Design review of the part built by this model. Coordinates are the model's own, in mm. A direction names the side the tool comes from. Coordinates: 2 decimals unless noted, no trailing zeros. Write each loop counter-clockwise with the first axis right and the second up, starting at its lowest first coordinate (ties: lowest second). Pieces come first, ordered by that corner, then holes. Notation, with made-up numbers: M 89,78 L 145,78 A15 ccw 145,85 Z; hole C -32,76 d3. An arc over 180 degrees is marked long. Write each question's results on one line, items separated by ' | '. Start each with the question number.
Autodesk Inventor part; units mm, degrees
ref_plane "YZ Plane" through (0, 0, 0) normal (1, 0, 0) x (0, 1, 0)
ref_plane "XZ Plane" through (0, 0, 0) normal (0, 1, 0) x (-1, 0, 0)
ref_plane "XY Plane" through (0, 0, 0) normal (0, 0, 1) x (1, 0, 0)
sketch "Sketch1" plane through (0, 0, 0) normal (0, 1, 0) x (-1, 0, 0)
  line L0 (0, 0) -> (628.65, 0)
  line L1 (628.65, 0) -> (628.65, 518.16)
  line L2 (628.65, 518.16) -> (0, 518.16)
  line L3 (0, 518.16) -> (0, 0)
  line L4 (0, 346.71) -> (50.8, 346.71)
  line L5 (50.8, 346.71) -> (50.8, 171.45)
  line L6 (50.8, 171.45) -> (0, 171.45)
  line L7 (0, 171.45) -> (0, 346.71)
  line L8 (628.65, 346.71) -> (577.85, 346.71)
  line L9 (577.85, 346.71) -> (577.85, 171.45)
  line L10 (577.85, 171.45) -> (628.65, 171.45)
  line L11 (628.65, 171.45) -> (628.65, 346.71)
  dimension "d0" = 628.65
  dimension "d1" = 518.16
  dimension "d2" = 50.8
  dimension "d3" = 50.8
  dimension "d4" = 171.45
  dimension "d5" = 171.45
  dimension "d6" = 171.45
  dimension "d7" = 171.45
extrude "Extrusion1" add sketch "Sketch1" along normal blind 3.048 contours L3 L6 L5 L4 L2 L1 L8 L9 L10 L0
sketch "Sketch2" plane through (0, 3.048, 0) normal (0, 1, 0) x (1, 0, 0)
  line L0 (-577.85, -171.45) -> (-469.9, -171.45)
  line L1 (-469.9, -171.45) -> (-469.9, -346.71)
  line L2 (-469.9, -346.71) -> (-577.85, -346.71)
  line L3 (-577.85, -346.71) -> (-577.85, -171.45)
  line L4 (-50.8, -346.71) -> (-158.75, -346.71)
  line L5 (-158.75, -346.71) -> (-158.75, -171.45)
  line L6 (-158.75, -171.45) -> (-50.8, -171.45)
  line L7 (-50.8, -171.45) -> (-50.8, -346.71)
  dimension "d10" = 107.95
  dimension "d11" = 107.95
extrude "Extrusion3" add sketch "Sketch2" along normal blind 76.2
sketch "Sketch3" plane through (0, 3.048, 0) normal (0, 1, 0) x (1, 0, 0)
  line L0 (-628.65, -346.71) -> (-628.65, -518.16)
  line L1 (0, -518.16) -> (0, -346.71)
  line L2 (-50.8, -346.71) -> (-158.75, -346.71)
  line L3 (0, -171.45) -> (0, 0)
  line L4 (-628.65, 0) -> (-628.65, -171.45)
  line L5 (-577.85, -171.45) -> (-469.9, -171.45)
  line L6 (-628.65, -422.91) -> (0, -422.91)
  line L7 (0, -422.91) -> (0, -435.61)
  line L8 (0, -435.61) -> (-628.65, -435.61)
  line L9 (-628.65, -435.61) -> (-628.65, -422.91)
  line L10 (-628.65, -82.55) -> (0, -82.55)
  line L11 (0, -82.55) -> (0, -95.25)
  line L12 (0, -95.25) -> (-628.65, -95.25)
  line L13 (-628.65, -95.25) -> (-628.65, -82.55)
  dimension "d16" = 12.7
  dimension "d17" = 12.7
  dimension "d18" = 76.2
  dimension "d19" = 76.2
extrude "Extrusion4" add sketch "Sketch3" along normal blind 63.5
equation "\"d3\" = d2"
equation "\"d5\" = d4"
equation "\"d6\" = d4"
equation "\"d7\" = d4"
properties part number "eboard"
Item 1: We need section A-A on y = 15.5. State the section outline as (x, z) points.
Item 2: We need section D-D on z = 486. State the section outline as (x, y) points, then the cut area to 3 significant figures.
Item 3: Wall thickness on L1, parallel to Z at x = -113, y = 45; L2, parallel to Z at x = -269, y = 32.5; L3, parallel to X at y = 36, z = 221.5: over which ranges is each line inside the solid? List them lowest first.
Item 4: Draft analysis for pull direction Z (two halves, no side actions). For faces 5 (the flat face through (-469.9, 41, 258)), 6 (the flat face through (-310, 34, 435.61)), 7 (the flat face through (-106, 79.248, 258)), state which applies: released by +Z, released by -Z, zero draft, split by the parting line, or undercut.
Item 5: Insertion check: pin 1 Ø10 at (y, z) = (40.5, 336) entering from +X; pin 2 Ø1.5 at (y, z) = (67, 293) entering from -X; pin 3 Ø1.5 at (x, y) = (-87, 20) entering from -Z. Each pin has a flat end and moves straight along its axis. Give the tip position at first contact, or say it passes through.
Item 6: For faces 1 (the flat face through (-310, 3.048, 42)), 2 (the flat face through (-319, 66.548, 429)), 3 (the flat face through (-50.8, 39, 260)), 4 (the flat face through (-523, 41, 346.71)), list the 3-axis set-ups (+Z, -Z, +X, -X, +Y, -Y) from which the entire face can be reached by the end or side of a thin tool; tool diameter is ignored.
Item 7: We need section B-B on z = 219. State the section outline as (x, y) points, then the cut area to 3 significant figures.
Item 8: We need section C-C on x = -168. State the section outline as (y, z) points.
Answer:
1) outline: M -628.65,82.55 L 0,82.55 L 0,95.25 L -628.65,95.25 Z; M -628.65,422.91 L 0,422.91 L 0,435.61 L -628.65,435.61 Z; M -577.85,171.45 L -469.9,171.45 L -469.9,346.71 L -577.85,346.71 Z; M -158.75,171.45 L -50.8,171.45 L -50.8,346.71 L -158.75,346.71 Z
2) outline: M -628.65,0 L 0,0 L 0,3.05 L -628.65,3.05 Z | area: 1,920 mm^2
3) L1: z = 82.55 to 95.25, 171.45 to 346.71, 422.91 to 435.61 | L2: z = 82.55 to 95.25, 422.91 to 435.61 | L3: x = -577.85 to -469.9, -158.75 to -50.8
4) face 5: undercut | face 6: released by +Z | face 7: zero draft
5) pin 1: stops at x = -50.8 | pin 2: stops at x = -577.85 | pin 3: stops at z = 82.55
6) face 1: -Z, +X, -X, +Y | face 2: +Z, +X, -X, +Y | face 3: +X, +Y, -Y | face 4: +X, -X, +Y
7) outline: M -577.85,0 L -50.8,0 L -50.8,79.25 L -158.75,79.25 L -158.75,3.05 L -469.9,3.05 L -469.9,79.25 L -577.85,79.25 Z | area: 18,100 mm^2
8) outline: M 0,0 L 3.05,0 L 3.05,82.55 L 66.55,82.55 L 66.55,95.25 L 3.05,95.25 L 3.05,422.91 L 66.55,422.91 L 66.55,435.61 L 3.05,435.61 L 3.05,518.16 L 0,518.16 Z
